Model file for the job. Use its own axes, mm. A direction names the side the tool comes from. Round coordinates to 2 decimals unless told otherwise and drop trailing zeros. Write each loop counter-clockwise with the first axis right and the second up, starting at its lowest first coordinate (ties: lowest second). Pieces come first, ordered by that corner, then holes. Notation, with made-up numbers: (53.25, -3) - (84.25, -3) arc R14 cw to (84.25, 18) - close; hole circle Ø4 at (26, 11.25). An arc over 180 degrees is marked (long way). One line per item, written item: value.
from build123d import *

# Parameters (mm, degrees)
SKETCH1_W           = 220
SKETCH1_H           = 220
SKETCH1_R           = 1.75
BOSS_EXTRUDE1_DEPTH = 15
FILLET1_R           = 10
BOSS_EXTRUDE2_DEPTH = 43
CUT_EXTRUDE1_DEPTH  = 31
FILLET2_R           = 2
SKETCH5_R           = 3.75
CUT_EXTRUDE2_DEPTH  = 4


with BuildPart() as part:
    # Sketch1 → Boss-Extrude1 (new body)
    with BuildSketch(Plane(origin=(0, 0, 0), x_dir=(1, 0, 0), z_dir=(0, 1, 0))):
        Rectangle(SKETCH1_W, SKETCH1_H)
        with Locations(Location((45.5, 15.5, 0), (0, 0, 270))):
            Circle(SKETCH1_R, mode=Mode.SUBTRACT)
        with Locations(Location((45.5, -15.5, 0), (0, 0, 90))):
            Circle(SKETCH1_R, mode=Mode.SUBTRACT)
        with Locations(Location((14.5, -15.5, 0), (0, 0, 270))):
            Circle(SKETCH1_R, mode=Mode.SUBTRACT)
        with Locations(Location((14.5, 15.5, 0), (0, 0, 90))):
            Circle(SKETCH1_R, mode=Mode.SUBTRACT)
    extrude(amount=BOSS_EXTRUDE1_DEPTH)

    # Fillet1
    fillet1_edges = [part.edges().sort_by_distance(p)[0] for p in [
        (110, 7.5, 110),
        (-110, 7.5, 110),
        (-110, 7.5, -110),
        (110, 7.5, -110),
    ]]
    fillet(fillet1_edges, radius=FILLET1_R)

    # Sketch2 → Boss-Extrude2 (add)
    with BuildSketch(Plane.XZ):
        with BuildLine():
            Line((-75, 95), (-85, 95))
            ThreePointArc((-85, 95), (-92.071067812, 92.071067812), (-95, 85))
            Line((-95, 85), (-95, 75))
            Line((-95, 75), (-110, 75))
            Line((-110, 75), (-110, 100))
            ThreePointArc((-110, 100), (-107.071067812, 107.071067812), (-100, 110))
            Line((-100, 110), (-75, 110))
            Line((-75, 110), (-75, 95))
        make_face()
        with BuildLine():
            Line((-75, -95), (-75, -110))
            Line((-75, -110), (-100, -110))
            ThreePointArc((-100, -110), (-107.071067812, -107.071067812), (-110, -100))
            Line((-110, -100), (-110, -75))
            Line((-110, -75), (-95, -75))
            Line((-95, -75), (-95, -85))
            ThreePointArc((-95, -85), (-92.071067812, -92.071067812), (-85, -95))
            Line((-85, -95), (-75, -95))
        make_face()
        with BuildLine():
            Line((75, -95), (85, -95))
            ThreePointArc((85, -95), (92.071067812, -92.071067812), (95, -85))
            Line((95, -85), (95, -75))
            Line((95, -75), (110, -75))
            Line((110, -75), (110, -100))
            ThreePointArc((110, -100), (107.071067812, -107.071067812), (100, -110))
            Line((100, -110), (75, -110))
            Line((75, -110), (75, -95))
        make_face()
        with BuildLine():
            Line((75, 95), (75, 110))
            Line((75, 110), (100, 110))
            ThreePointArc((100, 110), (107.071067812, 107.071067812), (110, 100))
            Line((110, 100), (110, 75))
            Line((110, 75), (95, 75))
            Line((95, 75), (95, 85))
            ThreePointArc((95, 85), (92.071067812, 92.071067812), (85, 95))
            Line((85, 95), (75, 95))
        make_face()
    extrude(amount=BOSS_EXTRUDE2_DEPTH)

    # Sketch3 → Cut-Extrude1 (cut)
    with BuildSketch(Plane.XZ.offset(43)):
        with BuildLine():
            ThreePointArc((-106.325, -85), (-100.079052109, -100.079052109), (-85, -106.325))
            ThreePointArc((-85, -106.325), (-81.675, -103), (-85, -99.675))
            ThreePointArc((-85, -99.675), (-95.376792014, -95.376792014), (-99.675, -85))
            ThreePointArc((-99.675, -85), (-103, -81.675), (-106.325, -85))
        make_face()
        with BuildLine():
            ThreePointArc((-85, 106.325), (-100.079052109, 100.079052109), (-106.325, 85))
            ThreePointArc((-106.325, 85), (-103, 81.675), (-99.675, 85))
            ThreePointArc((-99.675, 85), (-95.376792014, 95.376792014), (-85, 99.675))
            ThreePointArc((-85, 99.675), (-81.675, 103), (-85, 106.325))
        make_face()
        with BuildLine():
            ThreePointArc((106.325, 85), (100.079052109, 100.079052109), (85, 106.325))
            ThreePointArc((85, 106.325), (81.675, 103), (85, 99.675))
            ThreePointArc((85, 99.675), (95.376792014, 95.376792014), (99.675, 85))
            ThreePointArc((99.675, 85), (103, 81.675), (106.325, 85))
        make_face()
        with BuildLine():
            ThreePointArc((85, -106.325), (100.079052109, -100.079052109), (106.325, -85))
            ThreePointArc((106.325, -85), (103, -81.675), (99.675, -85))
            ThreePointArc((99.675, -85), (95.376792014, -95.376792014), (85, -99.675))
            ThreePointArc((85, -99.675), (81.675, -103), (85, -106.325))
        make_face()
    extrude(amount=-CUT_EXTRUDE1_DEPTH, mode=Mode.SUBTRACT)

    # Fillet2
    fillet2_edges = [part.edges().sort_by_distance(p)[0] for p in [
        (-75, -21.5, -95),
        (-95, -21.5, -75),
        (-110, -21.5, -75),
        (-75, -21.5, -110),
        (75, -21.5, 95),
        (95, -21.5, 75),
        (110, -21.5, 75),
        (75, -21.5, 110),
        (-110, -21.5, 75),
        (-95, -21.5, 75),
        (-75, -21.5, 95),
        (-75, -21.5, 110),
        (110, -21.5, -75),
        (95, -21.5, -75),
        (75, -21.5, -95),
        (75, -21.5, -110),
    ]]
    fillet(fillet2_edges, radius=FILLET2_R)

    # Sketch5 → Cut-Extrude2 (cut)
    with BuildSketch(Plane(origin=(0, 15, 0), x_dir=(1, 0, 0), z_dir=(0, 1, 0))):
        with Locations(Location((14.5, 15.5, 0), (0, 0, 270))):
            Circle(SKETCH5_R)
        with Locations(Location((45.5, 15.5, 0), (0, 0, 270))):
            Circle(SKETCH5_R)
        with Locations(Location((14.5, -15.5, 0), (0, 0, 270))):
            Circle(SKETCH5_R)
        with Locations(Location((45.5, -15.5, 0), (0, 0, 270))):
            Circle(SKETCH5_R)
    extrude(amount=-CUT_EXTRUDE2_DEPTH, mode=Mode.SUBTRACT)


solid = part.part
1. Band-saw the part on C-C on z = -25.5. Write the cut outline in (x, y), plus the area to 3 significant figures.
Report:
outline: (-110, 0) - (110, 0) - (110, 15) - (-110, 15) - close
area: 3,300 mm²
2. Band-saw the part on B-B on y = -5.5. State how many separate pieces and enclosed holes the cut face has, plus the area to 3 significant figures.
Report:
separate pieces: 4
enclosed holes: 0
area: 3,290 mm²
3. Wall check: probe 1 along X at (y, z) = (12.9, -15.5); probe 2 along Z at (x, y) = (45.5, 2.75); probe 3 along Z at (x, y) = (14, 12). Give the ranges that are in metal, low to high. Write a range as [from, to].
Report:
probe 1: [-110, 10.75], [18.25, 41.75], [49.25, 110]
probe 2: [-110, -17.25], [-13.75, 13.75], [17.25, 110]
probe 3: [-110, -19.22], [-11.78, 11.78], [19.22, 110]
4. Drop flat-ended pins along their axis: pin 1 (5 mm diameter, centred on x = -59, z = 13, fed in from -Y); pin 2 (4 mm diameter, centred on x = 44, z = -15, fed in from +Y); pin 3 (12 mm diameter, centred on y = -11.5, z = 43, fed in from +X); pin 4 (3.5 mm diameter, centred on x = 103.5, y = -21, fed in from -Z). Give the stop position or say it passes through.
Report:
pin 1: y = 0
pin 2: y = 11
pin 3: through
pin 4: z = -109.85
5. Band-saw the part on A-A on x = -103. Write the cut outline in (y, z) (3 decimals), plus the area to 3 significant figures.
Report:
outline: (-43, -109.539) - (15, -109.539) - (15, 109.539) - (-43, 109.539) - (-43, 96.435) - (-12, 96.435) - (-12, 81.675) - (-43, 81.675) - (-43, 75) - (0, 75) - (0, -75) - (-43, -75) - (-43, -81.675) - (-12, -81.675) - (-12, -96.435) - (-43, -96.435) - close
area: 5,340 mm²
6. Mould opens along X. For faces 1 (the face through (-75, -21, -102)), 2 (the face through (110, 5, 1)) say: released by +X, released by -X, zero draft, split by the parting line, or undercut.
Report:
face 1: undercut
face 2: released by +X
7. Band-saw the part on D-D on x = -30.5. Write the cut outline in (y, z), plus the area to 3 significant figures.
Report:
outline: (0, -110) - (15, -110) - (15, 110) - (0, 110) - close
area: 3,300 mm²
8. Tool access for faces 3 (the face through (10.84, 13.03, 14.69)), 4 (the face through (-95, -21, -81)): list every direction of +Z, -Z, +X, -X, +Y, -Y with a clear straight run to the whole face (end or side of a thin tool).
Report:
face 3: +Y
face 4: -Y
